Part print with two shaded views. Sizes in mm from the minimum x, y, z corner. Coordinates: 2 decimals unless noted, no trailing zeros. Loops run counter-clockwise (first coordinate to the right, second up) from the corner with the lowest first, then second, coordinate; pieces in that order, holes last. Notation, with made-up numbers: (76, -34) -> (131, -34) arc R23 cw to (131, -1) -> close; hole circle Ø5 at (34, 16.5). An arc over 180 degrees is marked (long way). Return JSON: item names as keys, results as strings. Group by question number.
(1) Saw through at A-A on y = 4.5. Write the cut outline in (x, z), then the cut area to 3 significant figures.
(2) Saw through at C-C on z = 7.5. Write the cut outline in (x, y), then the cut area to 3 significant figures.
(3) Saw through at B-B on x = 16.5. Write the cut outline in (y, z), then the cut area to 3 significant figures.
(4) Flat gauge pin, fed straight in: pin 1 Ø1 at (x, y) = (9.5, 2) entering from +Z. Where does the tip first touch, or does it go through?
(5) Saw through at D-D on x = 6.5. Write the cut outline in (y, z), then the cut area to 3 significant figures.
(6) Probe L1, parallel to Z at x = 18.5, y = 1.75; L2, parallel to Z at x = 12, y = 2.5; L3, parallel to X at y = 7.75, z = 4 (1 decimal). List the from-to ranges inside material, lowest first.
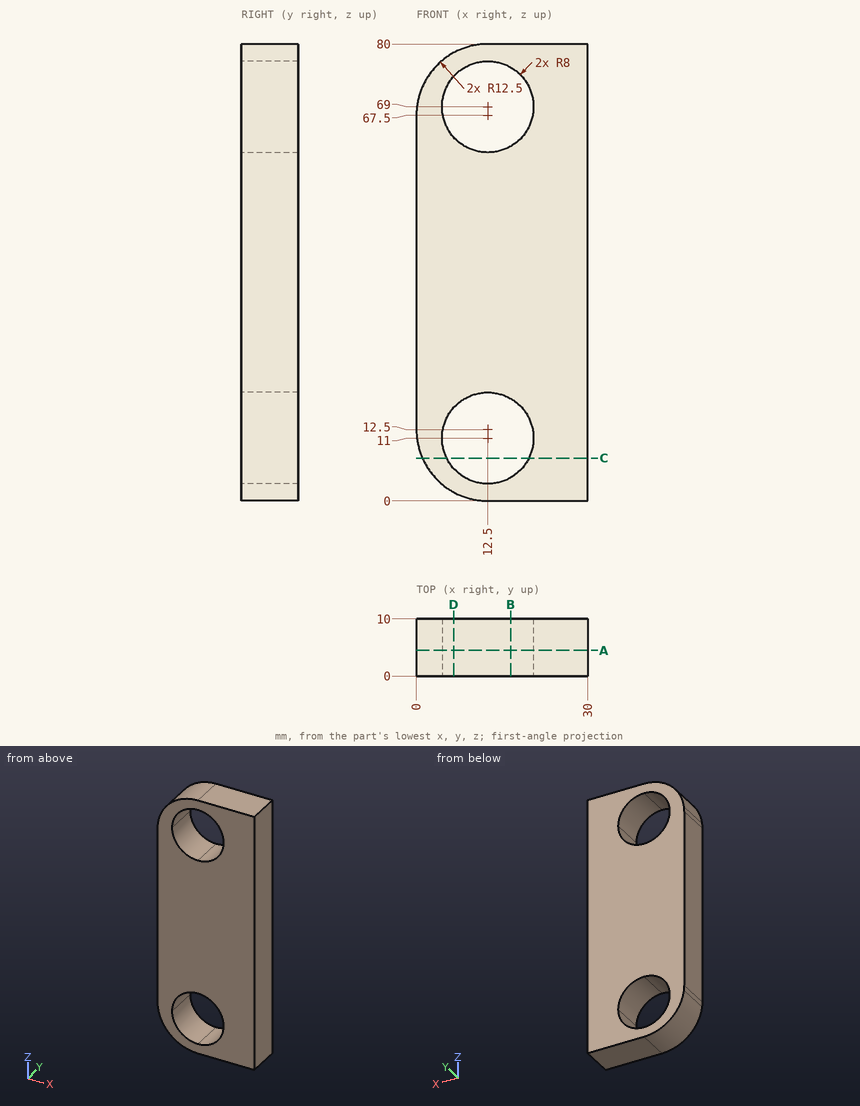
Geometry results:
{
 "1": {"outline": "(0, 12.5) arc R12.5 ccw to (0.09, 11) arc R12.5 ccw to (12.5, 0) -> (30, 0) -> (30, 80) -> (12.5, 80) arc R12.5 ccw to (0.09, 69) arc R12.5 ccw to (0, 67.5) -> close; hole (4.5, 11) arc R8 ccw to (12.5, 3) arc R8 ccw to (20.5, 11) arc R8 ccw to (12.5, 19) arc R8 ccw to start; hole (4.5, 69) arc R8 ccw to (12.5, 61) arc R8 ccw to (20.5, 69) arc R8 ccw to (12.5, 77) arc R8 ccw to start", "area": "1,930 mm²"},
 "2": {"outline": "(1.04, 0) -> (5.31, 0) -> (5.31, 10) -> (1.04, 10) -> close; (19.69, 0) -> (30, 0) -> (30, 10) -> (19.69, 10) -> close", "area": "146 mm²"},
 "3": {"outline": "(0, 0) -> (10, 0) -> (10, 4.07) -> (0, 4.07) -> close; (0, 17.93) -> (10, 17.93) -> (10, 62.07) -> (0, 62.07) -> close; (0, 75.93) -> (10, 75.93) -> (10, 80) -> (0, 80) -> close", "area": "523 mm²"},
 "4": {"pin 1": "z = 79.75"},
 "5": {"outline": "(0, 1.53) -> (10, 1.53) -> (10, 5.71) -> (0, 5.71) -> close; (0, 16.29) -> (10, 16.29) -> (10, 63.71) -> (0, 63.71) -> close; (0, 74.29) -> (10, 74.29) -> (10, 78.47) -> (0, 78.47) -> close", "area": "558 mm²"},
 "6": {"L1": "0 to 5.71, 16.29 to 63.71, 74.29 to 80", "L2": "0.01 to 3.02, 18.98 to 61.02, 76.98 to 79.99", "L3": "3.3 to 8.6, 16.4 to 30"}
}
